Build history of the part. All positions in model axes, mm. A direction names the side the tool comes from. Round coordinates to 2 decimals unless told otherwise and drop trailing zeros. Write each loop counter-clockwise with the first axis right and the second up, starting at its lowest first coordinate (ties: lowest second). Pieces come first, ordered by that corner, then holes. Notation, with made-up numbers: (-16.5, 32.25) - (39.5, 32.25) arc R30 cw to (39.5, 57.25) - close; hole circle Ø11 at (-13, -22). An arc over 180 degrees is marked (long way). Answer as a JSON object with one key per item and string values. Group by question number.
Item 1: Probe line 1 (X direction, y = 17.5, z = 2.5) (3 decimals); line 2 (Y direction, x = 99, z = 20.5) (3 decimals). List the from-to ranges inside material, lowest first. Write a range as from..to.
Item 2: Slice it at B-B, the plane z = 16.5. List the corners of the cut face in (x, y) (3 decimals), then the cut area to 3 significant figures.
Item 3: Which spindle directions (+Z, -Z, +X, -X, +Y, -Y) get a long thin tool onto all of the face, cutting with end or side? Do faces 1 (the flat face through (-5, 0, 13)), 2 (the flat face through (-5, 3.175, 14)). Say none if no direction does.
Item 4: Flat gauge pins, fed straight in: pin 1 (3.5 mm diameter, centred on y = 2, z = 10.5, fed in from +X); pin 2 (5.5 mm diameter, centred on x = 378.93, y = 16.93, fed in from +Z) (3 decimals); pin 3 (12 mm diameter, centred on x = -280, z = 19.5, fed in from -Y); pin 4 (12 mm diameter, centred on x = -165.5, z = 19, fed in from +Y) (3 decimals). Where does each tip first touch, or does it go through?
Item 5: Slice it at A-A, the plane x = 313.5. List the corners of the cut face in (y, z) (3 decimals).
Autodesk Inventor part; units mm, degrees
ref_plane "YZ Plane" through (0, 0, 0) normal (1, 0, 0) x (0, 1, 0)
ref_plane "XZ Plane" through (0, 0, 0) normal (0, 1, 0) x (-1, 0, 0)
ref_plane "XY Plane" through (0, 0, 0) normal (0, 0, 1) x (1, 0, 0)
sketch "Sketch1" plane through (0, 0, 0) normal (1, 0, 0) x (0, 1, 0)
  line L0 (25.4, 25.4) -> (0, 25.4) construction
  line L1 (0, 25.4) -> (0, 0)
  line L2 (0, 0) -> (25.4, 0)
  line L3 (25.4, 0) -> (25.4, 25.4) construction
  line L4 (25.4, 25.4) -> (3.175, 25.4) construction
  line L5 (3.175, 25.4) -> (3.175, 3.175)
  line L6 (3.175, 3.175) -> (25.4, 3.175)
  line L7 (25.4, 3.175) -> (25.4, 25.4) construction
  line L8 (25.4, 3.175) -> (25.4, 0)
  line L9 (3.175, 25.4) -> (0, 25.4)
  point P0 (0, 0)
  dimension "d1" = 25.4
  dimension "d2" = 3.175
extrude "Extrusion1" add sketch "Sketch1" along normal mid plane 781.15
sketch "Sketch2" plane through (-390.575, 3.175, 25.4) normal (0, 1, 0) x (1, 0, 0)
  line L0 (0, 0) -> (781.15, 0)
  line L1 (0, 0) -> (29.575, 0)
  line L2 (29.575, 0) -> (29.575, 22.225)
  line L3 (29.575, 22.225) -> (0, 22.225)
  line L4 (0, 22.225) -> (0, 0)
  line L5 (0, 22.225) -> (781.15, 22.225)
  point P0 (390.575, 25.4)
  point P1 (29.575, 0)
  dimension "d5" = 29.575
extrude "Extrusion2" cut sketch "Sketch2" against normal blind 3.175
sketch "Sketch3" plane through (-390.575, 25.4, 3.175) normal (0, 0, 1) x (1, 0, 0)
  line L0 (0, 0) -> (781.15, 0) construction
  line L1 (3.175, 0) -> (28.575, 0) construction
  line L2 (28.575, 0) -> (28.575, -25.4) construction
  line L3 (28.575, -25.4) -> (3.175, -25.4) construction
  line L4 (3.175, -25.4) -> (3.175, 0) construction
  line L5 (0, -25.4) -> (0, 0) construction
  line L6 (11.6417, -8.4667) -> (20.1083, -8.4667) construction
  line L7 (20.1083, -8.4667) -> (20.1083, -16.9333) construction
  line L8 (20.1083, -16.9333) -> (11.6417, -16.9333) construction
  line L9 (11.6417, -16.9333) -> (11.6417, -8.4667) construction
  circle A0 centre (11.6417, -8.4667) radius 2.4257
  circle A1 centre (20.1083, -16.9333) radius 2.4257
  point P0 (390.575, -25.4)
  point P1 (15.875, -8.4667)
  point P2 (15.875, 0)
  point P3 (20.1083, -12.7)
  point P4 (28.575, -12.7)
  dimension "d14" = 3.175
  dimension "d15" = 25.4
  dimension "d16" = 8.4667
  dimension "d17" = 4.8514
extrude "Extrusion4" cut sketch "Sketch3" against normal blind 3.175
mirror "Mirror2" about plane through (0, 0, 0) normal (1, 0, 0) of "Extrusion4", "Extrusion2"
equation "\"d3\" = beamXW"
equation "\"d17\" = rivetHoleD"
equation "\"shelfMargin\" = 1"
equation "\"beamXW\" = 781.15"
equation "\"s_t\" = 3.175"
equation "\"rivetD\" = 4.7625"
equation "\"rivetHoleD\" = 4.8514"
properties part number "beamX"
Geometry says:
{
 "1": {"line 1": "x = -390.575..-381.292, -376.575..376.575, 381.292..390.575", "line 2": "y = 0..3.175"},
 "2": {"outline": "(-361, 0) - (361, 0) - (361, 3.175) - (-361, 3.175) - close", "area": "2,290 mm^2"},
 "3": {"face 1": "+Z, -Z, +X, -X, -Y", "face 2": "+Z, +X, -X, +Y"},
 "4": {"pin 1": "stops at x = 361", "pin 2": "stops at z = 3.175", "pin 3": "stops at y = 0", "pin 4": "stops at y = 3.175"},
 "5": {"outline": "(0, 0) - (25.4, 0) - (25.4, 3.175) - (3.175, 3.175) - (3.175, 25.4) - (0, 25.4) - close"}
}
